```python
from build123d import *

# Parameters (mm, degrees)
BOSS_EXTRUDE1_DEPTH  = 10.16
CUT_EXTRUDE1_DEPTH   = 64.754
SKETCH3_R            = 1.4605
CUT_EXTRUDE2_DEPTH   = 6.35
BOSS_EXTRUDE2_DEPTH  = 2.54
MIRROR2_COPY_1_DEPTH = 2.54
SKETCH6_R            = 4.445
SKETCH6_R_2          = 1.4605
BOSS_EXTRUDE3_DEPTH  = 2.54


with BuildPart() as part:
    # Sketch1 → Boss-Extrude1 (new body)
    with BuildSketch(Plane.XY):
        Polygon((25.527, 0), (-25.527, 0), (-25.527, 28.702), (-31.877, 28.702), (-31.877, -2.54), (31.877, -2.54), (31.877, 28.702), (25.527, 28.702), align=None)
    extrude(amount=BOSS_EXTRUDE1_DEPTH)

    # Sketch2 → Cut-Extrude1 (cut, through all)
    with BuildSketch(Plane(origin=(31.877, 0, 0), x_dir=(0, 0, -1), z_dir=(1, 0, 0))):
        with BuildLine():
            Line((-6.35, 28.702), (-6.35, 1.867416652))
            ThreePointArc((-6.35, 1.867416652), (-5.803046326, 0.546953674), (-4.482583348, 0))
            Line((-4.482583348, 0), (0, 0))
            Line((0, 0), (0, 28.702))
            Line((0, 28.702), (-6.35, 28.702))
        make_face()
    extrude(amount=-CUT_EXTRUDE1_DEPTH, mode=Mode.SUBTRACT)

    # Sketch3 → Cut-Extrude2 (cut)
    with BuildSketch(Plane.XZ.offset(2.54)):
        with Locations((-19.05, 5.08)):
            Circle(SKETCH3_R)
        with Locations((19.05, 5.08)):
            Circle(SKETCH3_R)
    extrude(amount=-CUT_EXTRUDE2_DEPTH, mode=Mode.SUBTRACT)

    # Sketch5 → Boss-Extrude2 (add)
    with BuildSketch(Plane(origin=(0, 28.702, 0), x_dir=(1, 0, 0), z_dir=(0, 1, 0))):
        with BuildLine():
            Line((-31.75, -6.35), (-31.75, 3.81))
            ThreePointArc((-31.75, 3.81), (-28.575, 5.125128061), (-25.4, 3.81))
            Line((-25.4, 3.81), (-25.4, -6.35))
            Line((-25.4, -6.35), (-31.75, -6.35))
        make_face()
    boss_extrude2 = extrude(amount=-BOSS_EXTRUDE2_DEPTH)

    # Mirror1: Boss-Extrude2 across plane
    add(boss_extrude2.mirror(Plane(origin=(0, 19.7358, 0), x_dir=(0, 0, 1), z_dir=(0, -1, 0))))

    # Mirror2: Boss-Extrude2 across plane
    add(boss_extrude2.mirror(Plane(origin=(0, 0, 0), x_dir=(0, 0, 1), z_dir=(1, 0, 0))))

    # Mirror2 copy 1 sketch → Mirror2 copy 1 (add)
    with BuildSketch(Plane(origin=(0, 10.7696, 0), x_dir=(-1, 0, 0), z_dir=(0, -1, 0))):
        with BuildLine():
            Line((-31.75, -6.35), (-31.75, 3.81))
            ThreePointArc((-31.75, 3.81), (-28.575, 5.125128061), (-25.4, 3.81))
            Line((-25.4, 3.81), (-25.4, -6.35))
            Line((-25.4, -6.35), (-31.75, -6.35))
        make_face()
    extrude(amount=-MIRROR2_COPY_1_DEPTH)

    # Sketch6 → Boss-Extrude3 (add)
    with BuildSketch(Plane.XZ.offset(2.54)):
        with Locations((-19.05, 5.08)):
            Circle(SKETCH6_R)
        with Locations((-19.05, 5.08)):
            Circle(SKETCH6_R_2, mode=Mode.SUBTRACT)
        with Locations((19.05, 5.08)):
            Circle(SKETCH6_R)
        with Locations((19.05, 5.08)):
            Circle(SKETCH6_R_2, mode=Mode.SUBTRACT)
    extrude(amount=BOSS_EXTRUDE3_DEPTH)


solid = part.part
```
Can you work these out from the model? Positions are in its coordinate system, mm. A direction names the side the tool comes from. Coordinates: 2 decimals unless noted, no trailing zeros. Loops run counter-clockwise (first coordinate to the right, second up) from the corner with the lowest first, then second, coordinate; pieces in that order, holes last. Notation, with made-up numbers: M 63,-14 L 91,-14 A30 cw 91,10 Z; hole C 87,49 d11. An arc over 180 degrees is marked long. Put each result on its own line as item: value. Start each with the question number.
(1) Imagine slicing it at A-A on y = 3.5. List the corners of the cut face in (x, z) for me, and give its area (3 significant figures).
(2) I need wall thicknesses on probe 1 along Y at (x, z) = (28, 1.5); probe 2 along X at (y, z) = (7.5, 8.75); probe 3 along Z at (x, y) = (19, -4). Which ranges of each line are inside material? Lowest first, please.
(3) Imagine slicing it at B-B on x = -19.05. List the corners of the cut face in (y, z) for me (1 decimal), and give its area (3 significant figures).
(4) Imagine slicing it at C-C on z = 5.08. Give the number of separate pieces and of enclosed holes in the cut face, and give its area (3 significant figures).
(5) Which directions (+Z, -Z, +X, -X, +Y, -Y) give clear straight access to the entire face, cutting with the end or side of a thin tool? Please do faces 1 (the face through (0, -1, 0)), 2 (the face through (-31.75, 12, 1)), 3 (the face through (31.75, 27, 1)), 4 (the face through (29, 10.77, 1)), 5 (the face through (-25.4, 12, 1)).
(6) Imagine slicing it at D-D on x = -6. List the corners of the cut face in (y, z) for me, and give its area (3 significant figures).
(7) Will these pins go through, and if not, where does the flat tip stop? pin 1 Ø1.9 at (x, z) = (27.5, -1) entering from -Y; pin 2 Ø3 at (x, z) = (-6.5, 7) entering from +Y; pin 3 Ø2 at (x, y) = (19, 1.5) entering from -Z; pin 4 Ø3 at (y, z) = (12.5, -1) entering from -X.
Worked answers:
1. outline: M -31.88,6.35 L -25.53,6.35 L -25.53,10.16 L -31.88,10.16 Z; M 25.53,6.35 L 31.88,6.35 L 31.88,10.16 L 25.53,10.16 Z
1. area: 48.4 mm2
2. probe 1: y = -2.54 to 0, 10.77 to 13.31, 26.16 to 28.7
2. probe 2: x = -31.88 to -25.53, 25.53 to 31.88
2. probe 3: z = 0.64 to 3.62, 6.54 to 9.52
3. outline: M -5.1,0.6 L -2.5,0.6 L -2.5,0 L 0,0 L 0,3.6 L -5.1,3.6 Z; M -5.1,6.5 L 0,6.5 L 0,10.2 L -2.5,10.2 L -2.5,9.5 L -5.1,9.5 Z
3. area: 33.5 mm2
4. separate pieces: 7
4. enclosed holes: 0
4. area: 243 mm2
5. face 1: -Z, +X, -X, -Y
5. face 2: -Z, -X, +Y
5. face 3: -Z, +X, +Y
5. face 4: -Z, +X, -X
5. face 5: +Z, -Z, +Y
6. outline: M -2.54,0 L 0,0 L 0,10.16 L -2.54,10.16 Z
6. area: 25.8 mm2
7. pin 1: stops at y = 10.77
7. pin 2: stops at y = 0
7. pin 3: passes through
7. pin 4: stops at x = -31.75
